```python
from build123d import *

# Parameters (mm, degrees)
F0_R     = 3.175
F1_DEPTH = 40.64
F4_R     = 2.159
F5_DEPTH = 8.765794
F6_R     = 1.5875
F7_DEPTH = 12.7


with BuildPart() as f1:
    # F0 (on Front) → F1 (new body)
    with BuildSketch(Plane.XZ):
        Circle(F0_R)
    extrude(amount=F1_DEPTH)

    # F2 (on Top) → F3 (revolve, cut)
    with BuildSketch(Plane.XY):
        with BuildLine():
            Line((2.4847375462, -48.6786328256), (2.4847375462, -48.4504029155))
            Line((2.4847375462, -48.4504029155), (3.6910393974, -48.4504029155))
            Line((3.6910393974, -48.4504029155), (3.6910393974, -34.4593115151))
            Line((3.6910393974, -34.4593115151), (2.1464712918, -35.0223816931))
            ThreePointArc((2.1464712918, -35.0223816931), (1.8223472959, -35.5313199787), (2.1464712918, -36.0402582643))
            Line((2.1464712918, -36.0402582643), (2.8785056202, -36.3818742335))
            Line((2.8785056202, -36.3818742335), (2.4079122813, -37.009332329))
            Line((2.4079122813, -37.009332329), (1.121821173, -37.009332329))
            Line((1.121821173, -37.009332329), (1.121821173, -46.976801008))
            Line((1.121821173, -46.976801008), (2.4847375462, -48.6786328256))
        make_face()
    revolve(axis=Axis((0, -45.1813880354, 0), (0, 1, 0)), mode=Mode.SUBTRACT)

    # F4 (on Right) → F5 (join, symmetric)
    with BuildSketch(Plane.YZ):
        with Locations((-6.8540938167, 0)):
            Circle(F4_R)
    extrude(amount=F5_DEPTH, both=True)

    # F6 (on Right) → F7 (join, symmetric)
    with BuildSketch(Plane.YZ):
        with Locations((-6.8342058709, 0)):
            Circle(F6_R)
    extrude(amount=F7_DEPTH, both=True)


solid = f1.part
```
Work out the finished part from the listing and answer in its coordinate system (mm). A direction names the side the tool comes from. Give positions to 0.01 mm unless a question says otherwise; leave off trailing zeros. Write each loop counter-clockwise with the first axis right and the second up, starting at its lowest first coordinate (ties: lowest second). Pieces come first, ordered by that corner, then holes.
(1) Straight lines are drawn through the part: line 1 (Z direction, x = 2.75, y = -19.5); line 2 (Z direction, x = 0.25, y = -7.5). For each, find the intervals that lie inside material, in ascending order.
Final values:
line 1: z = -1.59 to 1.59
line 2: z = -3.17 to 3.17
(2) The part is cut by section A-A on x = 0. Write down the section's boundary in (y, z) (1 decimal), plus the area to 3 significant figures.
Final values:
outline: (-40.6, -1.1) - (-37, -1.1) - (-37, -2.4) - (-36.4, -2.9) - (-36, -2.1) arc R0.6 cw to (-35, -2.1) - (-34.6, -3.2) - (0, -3.2) - (0, 3.2) - (-34.6, 3.2) - (-35, 2.1) arc R0.6 cw to (-36, 2.1) - (-36.4, 2.9) - (-37, 2.4) - (-37, 1.1) - (-40.6, 1.1) - close
area: 239 mm2
(3) Flat-ended cylindrical pins translate along their axes: pin 1 Ø2 at (x, z) = (-7, -1) entering from -Y; pin 2 Ø2 at (y, z) = (-19.5, 0.5) entering from -X (3 decimals); pin 3 Ø1 at (y, z) = (-36.5, -2.5) entering from -X. Find the tip coordinate at first contact, or state that the pin passes through.
Final values:
pin 1: stops at y = -9.01
pin 2: stops at x = -3.175
pin 3: stops at x = -2.06
(4) The part is cut by section D-D on x = 7. Write down the section's boundary in (y, z), plus the area to 3 significant figures.
Final values:
outline: circle Ø4.32 at (-6.85, 0)
area: 14.6 mm2
(5) The part is cut by section C-C on y = -8. Write down the section's boundary in (x, z) (3 decimals).
Final values:
outline: (-12.7, -1.078) - (-8.766, -1.078) - (-8.766, -1.83) - (-2.595, -1.83) arc R3.175 ccw to (2.595, -1.83) - (8.766, -1.83) - (8.766, -1.078) - (12.7, -1.078) - (12.7, 1.078) - (8.766, 1.078) - (8.766, 1.83) - (2.595, 1.83) arc R3.175 ccw to (-2.595, 1.83) - (-8.766, 1.83) - (-8.766, 1.078) - (-12.7, 1.078) - close
(6) Which of the six approach directions +Z, -Z, +X, -X, +Y, -Y give full straight-line access (tool end or side, diameter ignored) to faces 1 (the flat face through (1, -37.009, 1)), 2 (the flat face through (-8.766, -7, 2)), 3 (the cylindrical face through (10.76, -8.42, 0.07)), 4 (the flat face through (0, -40.64, 0))?
Final values:
face 1: -Y
face 2: -X
face 3: +X
face 4: +Z, -Z, +X, -X, -Y
